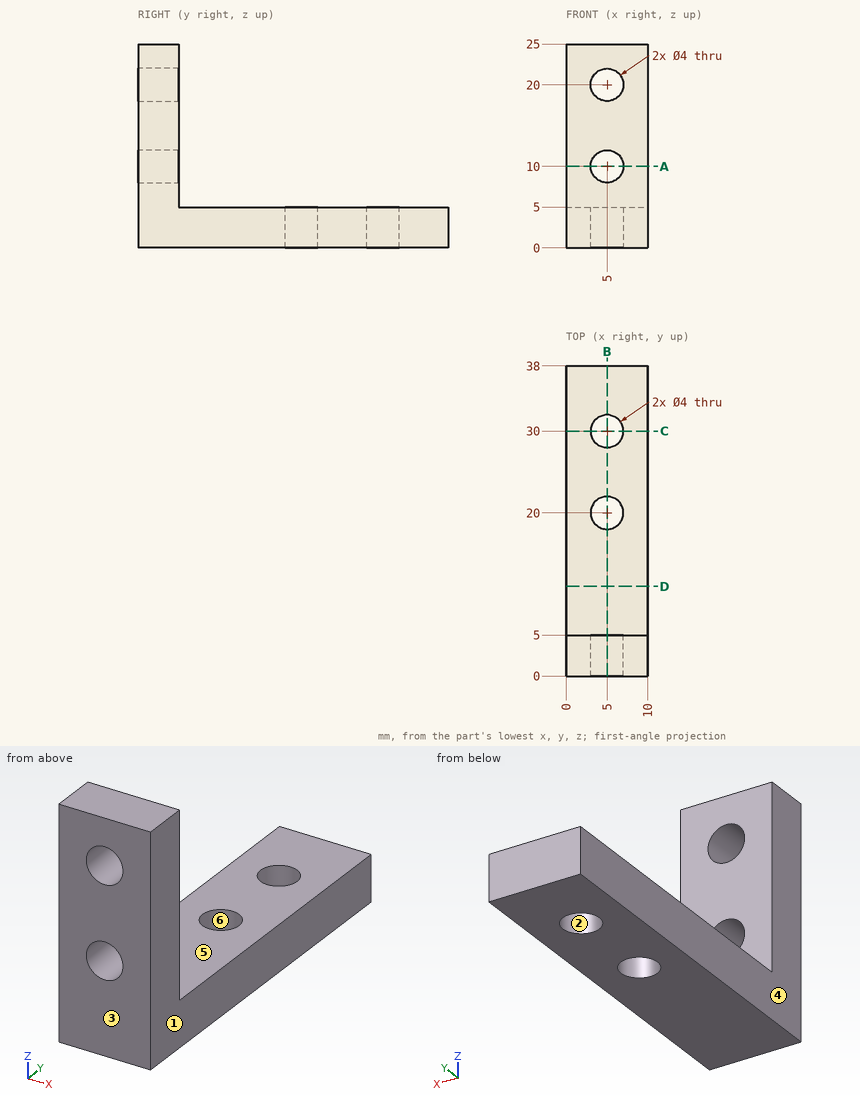
Geometry check sheet. Reference: drawing and pictorial views, mm from the part's lowest x, y, z. A direction names the side the tool comes from. Round coordinates to 2 decimals unless told otherwise and drop trailing zeros. Order: outer loops, then holes, each group sorted by start corner. A loop starts at its lowest first (then second) coordinate and runs counter-clockwise, first axis right, second up. Notation, with made-up numbers: M -15,-24 L 41,-24 A29 cw 41,12 Z; hole C -20,51.25 d6. An arc over 180 degrees is marked long. Write item = value, one per line.
Q1. Scan lines: line 1 (Z direction, x = 6.25, y = 4.5); line 2 (X direction, y = 1.25, z = 20); line 3 (Z direction, x = 2.75, y = 34). Record each from-to range of solid material in increasing order.
Answer block:
line_1 = 0 to 8.44, 11.56 to 18.44, 21.56 to 25
line_2 = 0 to 3, 7 to 10
line_3 = 0 to 5
Q2. Release check for a two-part mould opening along X. For the marked faces 1, 2, 3 and 4 record: released by +X, released by -X, zero draft, split by the parting line, or undercut.
Answer block:
face_1 = released by +X
face_2 = undercut
face_3 = zero draft
face_4 = released by -X
Q3. Section check B-B (x = 5). Enter the section's corners in (y, z), plus the area to 3 significant figures.
Answer block:
outline = M 0,0 L 18,0 L 18,5 L 5,5 L 5,8 L 0,8 Z; M 0,12 L 5,12 L 5,18 L 0,18 Z; M 0,22 L 5,22 L 5,25 L 0,25 Z; M 22,0 L 28,0 L 28,5 L 22,5 Z; M 32,0 L 38,0 L 38,5 L 32,5 Z
area = 210 mm^2
Q4. Depth check by flat-ended pin: pin 1 Ø3.5 at (x, z) = (5, 20) entering from -Y; pin 2 Ø3 at (x, z) = (6, 17) entering from +Y; pin 3 Ø2 at (x, y) = (2.5, 15) entering from +Z. Enter the tip coordinate at first touch or a pass-through.
Answer block:
pin_1 = through
pin_2 = 5
pin_3 = 5
Q5. Set-up check for the marked faces 5 and 6: record each of +Z, -Z, +X, -X, +Y, -Y from which the full face is reachable in a straight line by a thin tool's end or side.
Answer block:
face_5 = +Z, +X, -X, +Y
face_6 = +Z, -Z
Q6. Section check A-A (z = 10). Enter the section's corners in (x, y), plus the area to 3 significant figures.
Answer block:
outline = M 0,0 L 3,0 L 3,5 L 0,5 Z; M 7,0 L 10,0 L 10,5 L 7,5 Z
area = 30.0 mm^2
Q7. Section check D-D (y = 11). Enter the section's corners in (x, z), plus the area to 3 significant figures.
Answer block:
outline = M 0,0 L 10,0 L 10,5 L 0,5 Z
area = 50.0 mm^2
